from build123d import *

# Parameters (mm, degrees)
SKETCH2_W              = 19.1516
SKETCH2_H              = 10.9855
SKETCH2_R              = 2.31775
BOSS_EXTRUDE1_DEPTH    = 1.524
SKETCH3_W              = 9.6012
SKETCH3_H              = 1.7145
BOSS_EXTRUDE2_DEPTH    = 32.385
SKETCH4_W              = 9.6012
SKETCH4_H              = 19.05
BOSS_EXTRUDE3_DEPTH    = 9.271
SKETCH5_W              = 9.6012
SKETCH5_H              = 73.025
BOSS_EXTRUDE4_DEPTH    = 1.7145
SKETCH6_W              = 9.6012
SKETCH6_H              = 19.05
BOSS_EXTRUDE5_DEPTH    = 0.8509
SKETCH7_W              = 6.35
SKETCH7_H              = 21.844
BOSS_EXTRUDE6_DEPTH    = 0.508
BOSS_EXTRUDE7_DEPTH    = 0.508
SKETCH9_W              = 6.35
SKETCH9_H              = 31.75
BOSS_EXTRUDE8_DEPTH    = 0.508
SKETCH10_W             = 6.35
SKETCH10_H             = 21.844
BOSS_EXTRUDE9_DEPTH    = 0.508
SKETCH11_W             = 9.6012
SKETCH11_H             = 31.75
BOSS_EXTRUDE10_DEPTH   = 0.508
BOSS_EXTRUDE11_DEPTH   = 2.54
SKETCH13_R             = 2.794
BOSS_EXTRUDE12_DEPTH   = 0.762
SKETCH14_W             = 9.6012
SKETCH14_H             = 19.05
BOSS_EXTRUDE13_DEPTH   = 6.6675
BOSS_EXTRUDE14_DEPTH   = 0.508
BOSS_EXTRUDE15_DEPTH   = 0.508
BOSS_EXTRUDE16_DEPTH   = 0.508
SKETCH19_R             = 2.794
BOSS_EXTRUDE17_DEPTH   = 0.8382
BOSS_EXTRUDE17_2_DEPTH = 0.8382


with BuildPart() as part:
    # Sketch2 → Boss-Extrude1 (new body)
    with BuildSketch(Plane(origin=(0, 0, 0), x_dir=(1, 0, 0), z_dir=(0, 1, 0))):
        with Locations((0, 5.49275)):
            Rectangle(SKETCH2_W, SKETCH2_H)
        with Locations(Location((-4.73075, 5.08, 0), (0, 0, 270))):
            Circle(SKETCH2_R, mode=Mode.SUBTRACT)
        with Locations(Location((4.73075, 5.08, 0), (0, 0, 270))):
            Circle(SKETCH2_R, mode=Mode.SUBTRACT)
    extrude(amount=-BOSS_EXTRUDE1_DEPTH)

    # Sketch3 → Boss-Extrude2 (add)
    with BuildSketch(Plane(origin=(0, 0, 0), x_dir=(1, 0, 0), z_dir=(0, 1, 0))):
        with Locations((0, 11.84275)):
            Rectangle(SKETCH3_W, SKETCH3_H)
    extrude(amount=-BOSS_EXTRUDE2_DEPTH)


with BuildPart() as body_2:
    # Sketch4 → Boss-Extrude3 (new body)
    with BuildSketch(Plane(origin=(0, 0, -12.7), x_dir=(-1, 0, 0), z_dir=(0, 0, -1))):
        with Locations((0, -22.86)):
            Rectangle(SKETCH4_W, SKETCH4_H)
    extrude(amount=BOSS_EXTRUDE3_DEPTH)

    # Sketch7 → Boss-Extrude6 (add)
    with BuildSketch(Plane(origin=(0, 0, -14.2875), x_dir=(-1, 0, 0), z_dir=(0, 0, -1))):
        with Locations((0, -2.413)):
            Rectangle(SKETCH7_W, SKETCH7_H)
    extrude(amount=BOSS_EXTRUDE6_DEPTH)

    # Sketch15 → Boss-Extrude14 (add)
    with BuildSketch(Plane(origin=(0, 0, -14.7955), x_dir=(-1, 0, 0), z_dir=(0, 0, -1))):
        with BuildLine():
            Line((-4.8006, -32.385), (-6.279341549, -39.273723719))
            ThreePointArc((-6.279341549, -39.273723719), (-4.719076281, -41.686941549), (-2.305858451, -40.126676281))
            Line((-2.305858451, -40.126676281), (-0.644021101, -32.385))
            Line((-0.644021101, -32.385), (-4.8006, -32.385))
        make_face()
        with BuildLine():
            Line((-2.90018742, -37.751946457), (-3.300008934, -39.614516659))
            ThreePointArc((-3.300008934, -39.614516659), (-4.431204791, -40.345891003), (-5.162579136, -39.214695145))
            Line((-5.162579136, -39.214695145), (-4.762757622, -37.352124944))
            ThreePointArc((-4.762757622, -37.352124944), (-3.631561764, -36.620750599), (-2.90018742, -37.751946457))
        make_face(mode=Mode.SUBTRACT)
    extrude(amount=BOSS_EXTRUDE14_DEPTH)

    # Sketch17 → Boss-Extrude15 (add)
    with BuildSketch(Plane(origin=(0, 0, -18.288), x_dir=(-1, 0, 0), z_dir=(0, 0, -1))):
        with BuildLine():
            Line((4.8006, -32.385), (6.279341549, -39.273723719))
            ThreePointArc((6.279341549, -39.273723719), (4.719076281, -41.686941549), (2.305858451, -40.126676281))
            Line((2.305858451, -40.126676281), (0.644021101, -32.385))
            Line((0.644021101, -32.385), (4.8006, -32.385))
        make_face()
        with BuildLine():
            Line((2.90018742, -37.751946457), (3.300008934, -39.614516659))
            ThreePointArc((3.300008934, -39.614516659), (4.431204791, -40.345891003), (5.162579136, -39.214695145))
            Line((5.162579136, -39.214695145), (4.762757622, -37.352124944))
            ThreePointArc((4.762757622, -37.352124944), (3.631561764, -36.620750599), (2.90018742, -37.751946457))
        make_face(mode=Mode.SUBTRACT)
    extrude(amount=BOSS_EXTRUDE15_DEPTH)

    # Sketch18 → Boss-Extrude16 (add)
    with BuildSketch(Plane.XY.offset(-19.6723)):
        with BuildLine():
            Line((4.8006, -32.385), (6.279341549, -39.273723719))
            ThreePointArc((6.279341549, -39.273723719), (4.719076281, -41.686941549), (2.305858451, -40.126676281))
            Line((2.305858451, -40.126676281), (0.644021101, -32.385))
            Line((0.644021101, -32.385), (4.8006, -32.385))
        make_face()
        with BuildLine():
            Line((2.90018742, -37.751946457), (3.300008934, -39.614516659))
            ThreePointArc((3.300008934, -39.614516659), (4.431204791, -40.345891003), (5.162579136, -39.214695145))
            Line((5.162579136, -39.214695145), (4.762757622, -37.352124944))
            ThreePointArc((4.762757622, -37.352124944), (3.631561764, -36.620750599), (2.90018742, -37.751946457))
        make_face(mode=Mode.SUBTRACT)
    extrude(amount=BOSS_EXTRUDE16_DEPTH)


with BuildPart() as body_3:
    # Sketch5 → Boss-Extrude4 (new body)
    with BuildSketch(Plane(origin=(0, 0, -21.971), x_dir=(-1, 0, 0), z_dir=(0, 0, -1))):
        with Locations((0, 4.1275)):
            Rectangle(SKETCH5_W, SKETCH5_H)
    extrude(amount=BOSS_EXTRUDE4_DEPTH)


with BuildPart() as body_4:
    # Sketch6 → Boss-Extrude5 (new body)
    with BuildSketch(Plane(origin=(0, 0, -23.6855), x_dir=(-1, 0, 0), z_dir=(0, 0, -1))):
        with Locations((0, -22.86)):
            Rectangle(SKETCH6_W, SKETCH6_H)
    extrude(amount=BOSS_EXTRUDE5_DEPTH)


with BuildPart() as body_5:
    # Sketch8 → Boss-Extrude7 (new body)
    with BuildSketch(Plane(origin=(0, 0, -14.7955), x_dir=(-1, 0, 0), z_dir=(0, 0, -1))):
        with BuildLine():
            Line((4.7625, -13.335), (-4.7625, -13.335))
            Line((-4.7625, -13.335), (-4.7625, 20.066))
            ThreePointArc((-4.7625, 20.066), (0, 35.345573323), (4.7625, 20.066))
            Line((4.7625, 20.066), (4.7625, -13.335))
        make_face()
    extrude(amount=BOSS_EXTRUDE7_DEPTH)

    # Sketch12 → Boss-Extrude11 (add)
    with BuildSketch(Plane.XY.offset(-14.7955)):
        with BuildLine():
            Line((-16.51, 14.263573323), (16.51, 14.263573323))
            ThreePointArc((16.51, 14.263573323), (18.306051224, 15.007522099), (19.05, 16.803573323))
            Line((19.05, 16.803573323), (19.05, 37.123573323))
            ThreePointArc((19.05, 37.123573323), (18.306051224, 38.919624547), (16.51, 39.663573323))
            Line((16.51, 39.663573323), (-16.51, 39.663573323))
            ThreePointArc((-16.51, 39.663573323), (-18.306051224, 38.919624547), (-19.05, 37.123573323))
            Line((-19.05, 37.123573323), (-19.05, 16.803573323))
            ThreePointArc((-19.05, 16.803573323), (-18.306051224, 15.007522099), (-16.51, 14.263573323))
        make_face()
    extrude(amount=BOSS_EXTRUDE11_DEPTH)

    # Sketch13 → Boss-Extrude12 (add)
    with BuildSketch(Plane.XY.offset(-12.2555)):
        with Locations(Location((0, 26.963573323, 0), (0, 0, 180))):
            Circle(SKETCH13_R)
    extrude(amount=BOSS_EXTRUDE12_DEPTH)


with BuildPart() as body_6:
    # Sketch9 → Boss-Extrude8 (new body)
    with BuildSketch(Plane(origin=(0, 0, -17.78), x_dir=(-1, 0, 0), z_dir=(0, 0, -1))):
        with Locations((0, 2.54)):
            Rectangle(SKETCH9_W, SKETCH9_H)
    extrude(amount=BOSS_EXTRUDE8_DEPTH)


with BuildPart() as body_7:
    # Sketch10 → Boss-Extrude9 (new body)
    with BuildSketch(Plane(origin=(0, 0, -18.288), x_dir=(-1, 0, 0), z_dir=(0, 0, -1))):
        with Locations((0, -2.413)):
            Rectangle(SKETCH10_W, SKETCH10_H)
    extrude(amount=BOSS_EXTRUDE9_DEPTH)


with BuildPart() as body_8:
    # Sketch11 → Boss-Extrude10 (new body)
    with BuildSketch(Plane(origin=(0, 0, -19.6723), x_dir=(-1, 0, 0), z_dir=(0, 0, -1))):
        with Locations((0, 2.54)):
            Rectangle(SKETCH11_W, SKETCH11_H)
    extrude(amount=BOSS_EXTRUDE10_DEPTH)


with BuildPart() as body_9:
    # Sketch14 → Boss-Extrude13 (new body)
    with BuildSketch(Plane.XY.offset(-21.971)):
        with Locations((0, 29.083)):
            Rectangle(SKETCH14_W, SKETCH14_H)
    extrude(amount=BOSS_EXTRUDE13_DEPTH)


with BuildPart() as body_10:
    # Sketch19 → Boss-Extrude17 (new body)
    with BuildSketch(Plane(origin=(0, 0, -24.5364), x_dir=(-1, 0, 0), z_dir=(0, 0, -1))):
        with Locations((0, -17.93875)):
            Circle(SKETCH19_R)
    extrude(amount=BOSS_EXTRUDE17_DEPTH)


with BuildPart() as body_11:
    # Sketch19 → Boss-Extrude17 2 (new body)
    with BuildSketch(Plane(origin=(0, 0, -24.5364), x_dir=(-1, 0, 0), z_dir=(0, 0, -1))):
        with Locations((0, -27.78125)):
            Circle(SKETCH19_R)
    extrude(amount=BOSS_EXTRUDE17_2_DEPTH)


with BuildPart() as part_1:
    add(part.part)

    # Combine1: union body 3, body 4, body 6, body 7, body 8, body 5, body 9, body 2, body 10, body 11
    add(body_3.part)
    add(body_4.part)
    add(body_6.part)
    add(body_7.part)
    add(body_8.part)
    add(body_5.part)
    add(body_9.part)
    add(body_2.part)
    add(body_10.part)
    add(body_11.part)


solid = part_1.part
Design review of the part built by this model. Coordinates are the model's own, in mm. A direction names the side the tool comes from. Coordinates: 2 decimals unless noted, no trailing zeros. Loops run counter-clockwise (first coordinate to the right, second up) from the corner with the lowest first, then second, coordinate; pieces in that order, holes last.
Item 1: For faces 4 (the flat face through (4, -36, -19.672)), 5 (the flat face through (7, -1, -10.986)), 6 (the flat face through (0, -13.335, -21)), 7 (the flat face through (0, -1.524, -6)), list the 3-axis set-ups (+Z, -Z, +X, -X, +Y, -Y) from which the entire face can be reached by the end or side of a thin tool; tool diameter is ignored.
Completed:
face 4: -Z, +X, -X, -Y
face 5: -Z, +X, +Y, -Y
face 6: +X, -X
face 7: +Z, +X, -X, -Y
Item 2: Add section C-C (y = -12). Write out the cut boundary in (x, z) (1 decimal), and give its area (3 significant figures).
Completed:
outline: (-4.8, -23.7) - (4.8, -23.7) - (4.8, -22) - (-4.8, -22) - close; (-4.8, -20.2) - (4.8, -20.2) - (4.8, -19.7) - (-4.8, -19.7) - close; (-4.8, -15.3) - (4.8, -15.3) - (4.8, -14.8) - (3.2, -14.8) - (3.2, -14.3) - (-3.2, -14.3) - (-3.2, -14.8) - (-4.8, -14.8) - close; (-4.8, -12.7) - (4.8, -12.7) - (4.8, -11) - (-4.8, -11) - close; (-3.2, -18.8) - (3.2, -18.8) - (3.2, -17.8) - (-3.2, -17.8) - close
area: 52.3 mm2
Item 3: Wall thickness on L1, parallel to X at y = -1, z = -5.08; L2, parallel to Y at x = -3, z = -16.75 (3 decimals); L3, parallel to Z at x = -10, y = 26: over which ranges is each line inside the solid? List them lowest first.
Completed:
L1: x = -9.58 to -7.05, -2.41 to 2.41, 7.05 to 9.58
L2: y = -32.385 to -13.335, 19.558 to 38.608
L3: z = -14.8 to -12.26
Item 4: Add section A-A (y = 6.5). Write out the cut boundary in (x, z) (1 decimal).
Completed:
outline: (-4.8, -23.7) - (4.8, -23.7) - (4.8, -22) - (-4.8, -22) - close; (-4.8, -20.2) - (4.8, -20.2) - (4.8, -19.7) - (-4.8, -19.7) - close; (-4.8, -15.3) - (4.8, -15.3) - (4.8, -14.8) - (3.2, -14.8) - (3.2, -14.3) - (-3.2, -14.3) - (-3.2, -14.8) - (-4.8, -14.8) - close; (-3.2, -18.8) - (3.2, -18.8) - (3.2, -17.8) - (-3.2, -17.8) - close
Item 5: Clearance check with flat-ended pins moving along their axes: pin 1 (1.4 mm diameter, centred on x = 1, z = -21, fed in from +Y); pin 2 (5.5 mm diameter, centred on x = 1.5, z = -17.5, fed in from -Y); pin 3 (2 mm diameter, centred on x = 3.5, y = 8, fed in from -Z). State where each tip first meets the part, or that it passes through.
Completed:
pin 1: stops at y = 38.61
pin 2: stops at y = -41.64
pin 3: stops at z = -23.69
Item 6: Add section D-D (z = -13.5). Write out the cut boundary in (x, y) (3 decimals), and give its area (3 significant figures).
Completed:
outline: (-19.05, 16.804) arc R2.54 ccw to (-16.51, 14.264) - (16.51, 14.264) arc R2.54 ccw to (19.05, 16.804) - (19.05, 37.124) arc R2.54 ccw to (16.51, 39.664) - (-16.51, 39.664) arc R2.54 ccw to (-19.05, 37.124) - close; (-4.801, -32.385) - (4.801, -32.385) - (4.801, -13.335) - (-4.801, -13.335) - close
area: 1,150 mm2
Item 7: Add section B-B (z = -5.08). Write out the cut boundary in (x, y).
Completed:
outline: (-9.58, -1.52) - (-7.05, -1.52) - (-7.05, 0) - (-9.58, 0) - close; (-2.41, -1.52) - (2.41, -1.52) - (2.41, 0) - (-2.41, 0) - close; (7.05, -1.52) - (9.58, -1.52) - (9.58, 0) - (7.05, 0) - close
Item 8: Draft analysis for pull direction Z (two halves, no side actions). For faces 1 (the flat face through (0, -23, -24.536)), 2 (the flat face through (0, -13.335, -16)), 3 (the flat face through (0, -17, -10.986)), state which applies: pulls with the +Z half, pulls with the -Z half, needs draft (parallel to the pull), parting line crosses it, or undercut.
Completed:
face 1: pulls with the -Z half
face 2: undercut
face 3: pulls with the +Z half
